Build history of the part. All positions in model axes, mm. A direction names the side the tool comes from. Give positions to 0.01 mm unless a question says otherwise; leave off trailing zeros. Order: outer loops, then holes, each group sorted by start corner. A loop starts at its lowest first (then second) coordinate and runs counter-clockwise, first axis right, second up. Notation, with made-up numbers: (-38.5, 8.25) - (2.5, 8.25) arc R18 cw to (2.5, 41.25) - close; hole circle Ø1 at (72, -30.5). An arc over 180 degrees is marked (long way). Answer in a Markdown table with one row per item.
```python
from build123d import *

# Parameters (mm, degrees)
ESBO_O1_R                = 4
RESSALTO_EXTRUS_O1_DEPTH = 4.5
ESBO_O3_R                = 4
RESSALTO_EXTRUS_O2_DEPTH = 2.5
ESBO_O5_R                = 2.4
CORTE_EXTRUS_O1_DEPTH    = 3.5


with BuildPart() as part:
    # Esbo_o1 → Ressalto-extrus_o1 (new body)
    with BuildSketch(Plane.XY):
        with Locations((25, 0.5)):
            Circle(ESBO_O1_R)
        with BuildLine():
            ThreePointArc((-5, -0.5), (-2.217514421, -7.217514421), (4.5, -10))
            Line((4.5, -10), (8.963244058, -10))
            ThreePointArc((8.963244058, -10), (9.978406451, -9.895860018), (10.951281246, -9.587778127))
            Line((10.951281246, -9.587778127), (25, -3.5))
            ThreePointArc((25, -3.5), (21, 0.5), (25, 4.5))
            Line((25, 4.5), (10.833504783, 9.694381579))
            ThreePointArc((10.833504783, 9.694381579), (9.986328816, 9.923002534), (9.112231538, 10))
            Line((9.112231538, 10), (4.5, 10))
            ThreePointArc((4.5, 10), (-2.217514421, 7.217514421), (-5, 0.5))
            Line((-5, 0.5), (-5, -0.5))
        make_face()
    extrude(amount=RESSALTO_EXTRUS_O1_DEPTH)

    # Esbo_o3 → Ressalto-extrus_o2 (add)
    with BuildSketch(Plane.XY.offset(4.5)):
        with Locations(Location((25, 0.5, 0), (0, 0, 90))):
            Circle(ESBO_O3_R)
    extrude(amount=RESSALTO_EXTRUS_O2_DEPTH)

    # Esbo_o5 → Corte-extrus_o1 (cut)
    with BuildSketch(Plane.XY.offset(7)):
        with Locations((25, 0.5)):
            Circle(ESBO_O5_R)
    extrude(amount=-CORTE_EXTRUS_O1_DEPTH, mode=Mode.SUBTRACT)


solid = part.part
```
1. Drop flat-ended pins along their axis: P1, Ø10, axis at x = 10, y = 1.5, coming from the +Z side; P2, Ø3, axis at y = -4.5, z = 5, coming from the -X side; P3, Ø1.4, axis at x = 24.5, y = 0, coming from the +Z side. Give the stop position or say it passes through.
Check result:
| item | result |
|---|---|
| P1 | stops at z = 4.5 |
| P2 | stops at x = -4.64 |
| P3 | stops at z = 3.5 |
2. Which spindle directions (+Z, -Z, +X, -X, +Y, -Y) get a long thin tool onto all of the face, cutting with end or side? Do faces 4 (the face through (-2.143, 7.291, 2.218)), 5 (the face through (27.29, 1.22, 5.27)). Say none if no direction does.
Check result:
| item | result |
|---|---|
| face 4 | +Z, -Z, -X, +Y |
| face 5 | +Z |
3. Cut at C-C on y = -6. Write the cut outline in (x, z), and give its area (3 significant figures).
Check result:
| item | result |
|---|---|
| outline | (-3.25, 0) - (19.23, 0) - (19.23, 4.5) - (-3.25, 4.5) - close |
| area | 101 mm² |
4. Probe line 1 (Y direction, x = 25, z = 5.9); line 2 (Z direction, x = 3.5, y = 3.25); line 3 (Z direction, x = 25, y = 2.25). List the from-to ranges inside material, lowest first.
Check result:
| item | result |
|---|---|
| line 1 | y = -3.5 to -1.9, 2.9 to 4.5 |
| line 2 | z = 0 to 4.5 |
| line 3 | z = 0 to 3.5 |
5. Two-plate mould, pull along X, no slides. Class faces 1 (the face through (18.02, 7.06, 2.22)), 2 (the face through (25, 1, 3.5)), 3 (the face through (10, 0, 4.5)): +X half, -X half, draft (parallel to the pull), parting line (faces both ways), or undercut.
Check result:
| item | result |
|---|---|
| face 1 | +X half |
| face 2 | undercut |
| face 3 | draft |
6. Cut at A-A on z = 5.75. Write the cut outline in (x, y).
Check result:
| item | result |
|---|---|
| outline | circle Ø8 at (25, 0.5); hole circle Ø4.8 at (25, 0.5) |
7. Cut at B-B on x = 15.5. Write the cut outline in (y, z), and give its area (3 significant figures).
Check result:
| item | result |
|---|---|
| outline | (-7.62, 0) - (7.98, 0) - (7.98, 4.5) - (-7.62, 4.5) - close |
| area | 70.2 mm² |
